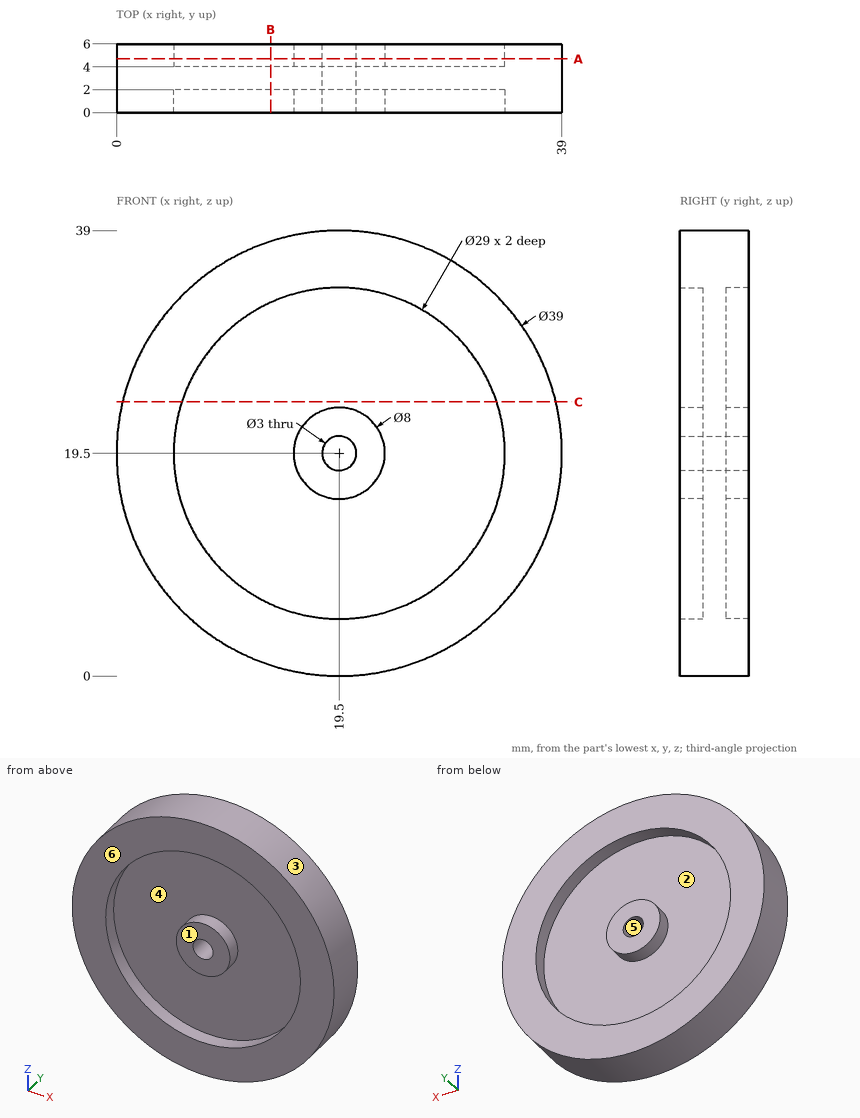
The drawing under review shows one solid part. Ordinate dimensions are in mm from its lowest x, y, z. A direction names the side the tool comes from. Coordinates: 2 decimals unless noted, no trailing zeros. Order: outer loops, then holes, each group sorted by start corner. A loop starts at its lowest first (then second) coordinate and runs counter-clockwise, first axis right, second up. Notation, with made-up numbers: M -18.75,87 L 31.25,87 A15 cw 31.25,97 Z; hole C -27,71.5 d4. An arc over 180 degrees is marked long. One line per question, with ' | ' between items.
(1) Add section C-C, the plane z = 24. Write out the cut boundary in (x, y), then the cut area to 3 significant figures.
Geometry results:
outline: M 0.53,0 L 5.72,0 L 5.72,2 L 33.28,2 L 33.28,0 L 38.47,0 L 38.47,6 L 33.28,6 L 33.28,4 L 5.72,4 L 5.72,6 L 0.53,6 Z | area: 117 mm²
(2) The part is to be moulded in two halves that separate along Z. For the marked faces 3, 4, 5 and 6, say which applies: +Z half, -Z half, draft (parallel to the pull), parting line (faces both ways), or undercut.
Geometry results:
face 3: parting line | face 4: undercut | face 5: undercut | face 6: draft
(3) For probe 1 along Z at (x, y) = (23, 0.8); probe 2 along Z at (x, y) = (20.5, 0.4) (1 decimal); probe 3 along Y at (x, z) = (12, 22), list the stretches that pass through material, from the lowest coordinate up. Write a range as from..to.
Geometry results:
probe 1: z = 0.32..5.43, 17.56..21.44, 33.57..38.68 | probe 2: z = 0..5, 15.6..18.4, 20.6..23.4, 34..39 | probe 3: y = 2..4
(4) Add section B-B, the plane x = 13.5. Write out the cut boundary in (y, z), then the cut area to 3 significant figures.
Geometry results:
outline: M 0,0.95 L 6,0.95 L 6,6.3 L 4,6.3 L 4,32.7 L 6,32.7 L 6,38.05 L 0,38.05 L 0,32.7 L 2,32.7 L 2,6.3 L 0,6.3 Z | area: 117 mm²
(5) Add section A-A, the plane y = 4.7. Write out the cut boundary in (x, z).
Geometry results:
outline: C 19.5,19.5 d39; C 19.5,19.5 d8; hole C 19.5,19.5 d29; hole C 19.5,19.5 d3
(6) Insertion check: pin 1 (1.8 mm diameter, centred on x = 19.5, z = 19.5, fed in from -Y); pin 2 (4 mm diameter, centred on x = 28.5, z = 25, fed in from -Y); pin 3 (2 mm diameter, centred on x = 5.5, y = 2.5, fed in from +Z); pin 4 (2 mm diameter, centred on x = 8.5, z = 25.5, fed in from +Y). Each pin has a flat end and moves straight along its axis. Give the tip position at first contact, or say it passes through.
Geometry results:
pin 1: passes through | pin 2: stops at y = 2 | pin 3: stops at z = 34.03 | pin 4: stops at y = 4
(7) Machinability: for the marked faces 1 and 2, which of the approach directions +Z, -Z, +X, -X, +Y, -Y give a long, thin tool a straight path to every point of the face, cutting with its end or side? Answer none if there is none.
Geometry results:
face 1: +Z, -Z, +X, -X, -Y | face 2: +Y
